Verification items for the finished model (mm, model axes). Give positions to 0.01 mm unless a question says otherwise; leave off trailing zeros. Order: outer loops, then holes, each group sorted by start corner. A loop starts at its lowest first (then second) coordinate and runs counter-clockwise, first axis right, second up.
(1) Scan lines: L1, parallel to Y at x = 0.15, z = 4 (3 decimals); L2, parallel to X at y = 0.9, z = 3.5 (3 decimals); L3, parallel to Y at x = 0.1, z = 16.5. Record each from-to range of solid material in increasing order.
(2) Sectioned sample at A-A on z = 20.75. Record the cut outline in (x, y).
(3) Gauge pin test, flat ends, axial feed: pin 1 (0.7 mm diameter, centred on x = 0.5, z = 3.5, fed in from +Y) (3 decimals); pin 2 (2 mm diameter, centred on y = 1.5, z = 12, fed in from -X). Record the tip position at first contact, or that the pin passes through.
(4) Mould release check, pull along Y, two halves, no side actions. Record for faces 1 (the face through (0, 1.175, 2)), 2 (the face through (0, -1.5, 0)), 3 (the face through (-0.29, 2.23, 10.35)): pulls with the +Y half, pulls with the -Y half, needs draft (parallel to the pull), parting line crosses it, or undercut.
```python
from build123d import *

# Parameters (mm, degrees)
SKETCH_1_R          = 2.25
EXTRUDE_2_DEPTH     = 23
SKETCH_7_W          = 2.35
SKETCH_7_H          = 2.35
CUT_EXTRUDE_3_DEPTH = 4.5
FILLET_2_R          = 2


with BuildPart() as part:
    # 草图1 → 凸台-拉伸2 (new body)
    with BuildSketch(Plane.XY):
        Circle(SKETCH_1_R)
    extrude(amount=EXTRUDE_2_DEPTH)

    # 草图7 → 切除-拉伸3 (cut)
    with BuildSketch(Plane.XY):
        Rectangle(SKETCH_7_W, SKETCH_7_H)
    extrude(amount=CUT_EXTRUDE_3_DEPTH, mode=Mode.SUBTRACT)

    # 圆角2
    fillet_2_edges = [part.edges().sort_by_distance(p)[0] for p in [
        (-2.25, 0, 23),
    ]]
    fillet(fillet_2_edges, radius=FILLET_2_R)


solid = part.part
```
Ans:
1. L1: y = -2.245 to -1.175, 1.175 to 2.245
1. L2: x = -2.062 to -1.175, 1.175 to 2.062
1. L3: y = -2.25 to 2.25
2. outline: circle Ø4.5 at (0, 0)
3. pin 1: stops at y = 2.245
3. pin 2: stops at x = -2.19
4. face 1: undercut
4. face 2: needs draft
4. face 3: parting line crosses it
